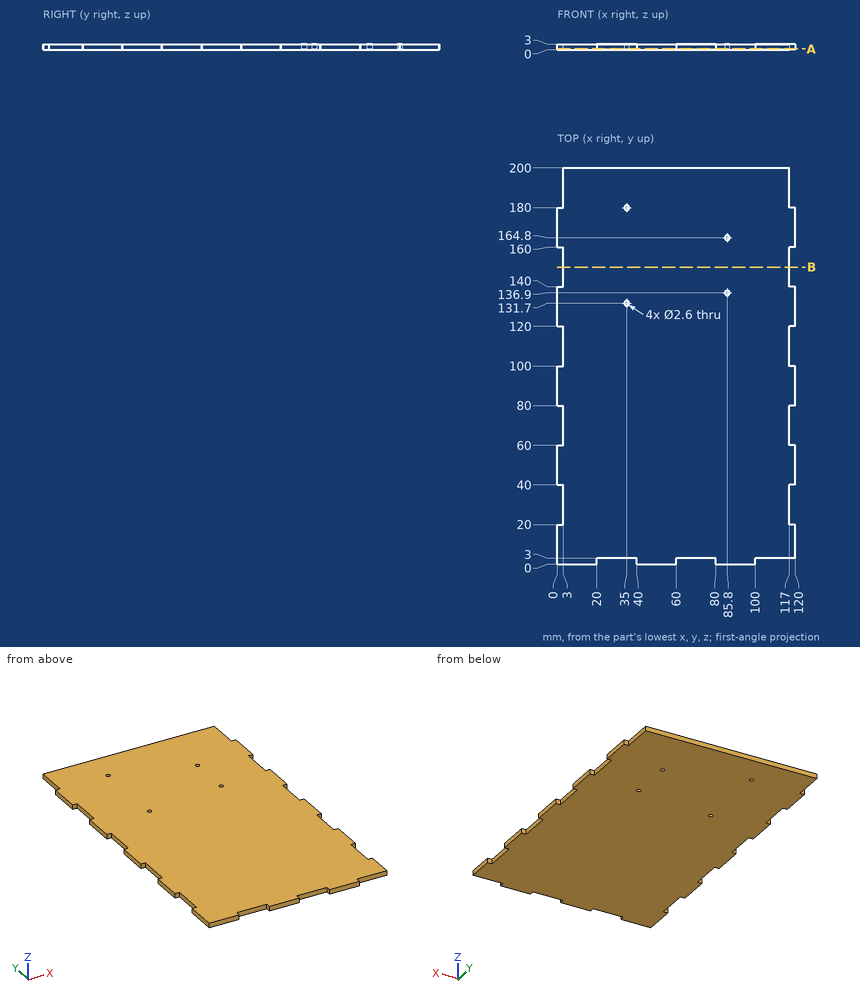
Study the drawing (mm; zero at the part's minimum x, y, z) and answer. Round coordinates to 2 decimals unless told otherwise and drop trailing zeros. Loops run counter-clockwise (first coordinate to the right, second up) from the corner with the lowest first, then second, coordinate; pieces in that order, holes last. Notation, with made-up numbers: (-16, -9.75) - (17, -9.75) arc R24 cw to (17, 15.25) - close; hole circle Ø8 at (56, 39). An arc over 180 degrees is marked (long way). Use one line per item in the form item = value. Start each with the question number.
1. Given pin 1 Ø0.9 at (y, z) = (30, 1.5) entering from +X; pin 2 Ø0.9 at (x, z) = (1, 2) entering from +Y; pin 3 Ø1.5 at (y, z) = (1, 1) entering from +X, each flat-ended and moving along its own axis, determine where each tip first touches the part or whether it passes through.
2. The part is cut by section B-B on y = 150. Determine the outline of the cut face in (x, z).
3. The part is cut by section A-A on z = 0.6. Give the number of separate pieces and of enclosed holes in the cut face, then the cut area to 3 significant figures.
4. Consider line 1 (Y direction, x = 35, z = 1.6); line 2 (Y direction, x = 85.8, z = 1.3); line 3 (X direction, y = 71.5, z = 2.2). Determine where each line is inside the solid, lowest interval first. Write a range as [from, to].
Geometry check:
q1.pin_1 = 117
q1.pin_2 = 180
q1.pin_3 = 100
q2.outline = (3, 0) - (117, 0) - (117, 3) - (3, 3) - close
q3.separate_pieces = 1
q3.enclosed_holes = 4
q3.area = 23,200 mm^2
q4.line_1 = [3, 130.4], [133, 178.7], [181.3, 200]
q4.line_2 = [0, 135.6], [138.2, 163.5], [166.1, 200]
q4.line_3 = [3, 117]
